Can you work these out from the drawing? Everything is in mm from the part's minimum corner. A direction names the side the tool comes from. Round coordinates to 2 decimals unless told otherwise and drop trailing zeros. Write each loop counter-clockwise with the first axis right and the second up, starting at its lowest first coordinate (ties: lowest second). Pieces come first, ordered by that corner, then holes. Notation, with made-up numbers: (51.5, -25.75) -> (75.5, -25.75) arc R9 ccw to (75.5, -9.75) -> close; hole circle Ø11 at (5.25, -14). An arc over 180 degrees is marked (long way). Write item = value, one per line. Start each with the question number.
1) Imagine slicing it at B-B, the plane x = 75. Please give me the cut outline in (y, z) (1 decimal).
2) Imagine slicing it at C-C, the plane y = 5.5. Please give me the cut outline in (x, z), then the cut area to 3 significant figures.
3) For the marked faces 1 and 2, which set-ups out of +Z, -Z, +X, -X, +Y, -Y let a thin tool reach every point of the face, with its end or its side?
4) Imagine slicing it at A-A, the plane z = 8. Please give me the cut outline in (x, y) (1 decimal).
5) If I drill on line 1 (Y direction, x = 52, z = 19) (1 decimal); line 2 (Z direction, x = 88.5, y = 21.5) (1 decimal); line 3 (Z direction, x = 17, y = 22), over which ranges is the centre line in solid material (lowest first)?
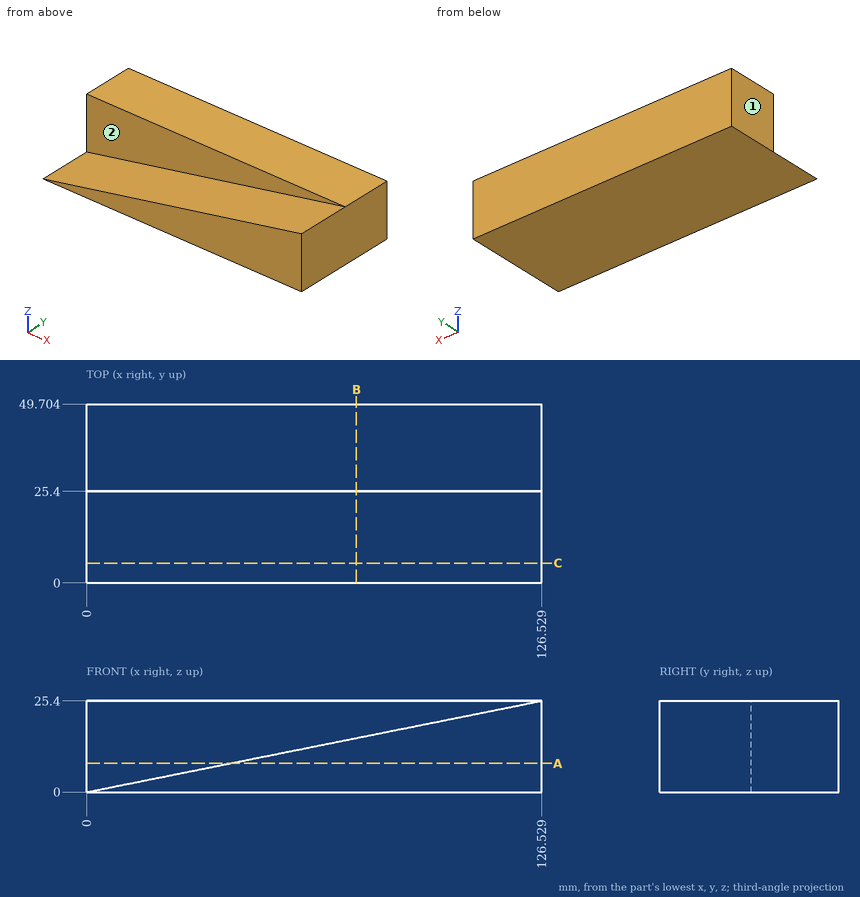
Reported:
q1.outline = (0, 0) -> (49.7, 0) -> (49.7, 25.4) -> (25.4, 25.4) -> (25.4, 15.1) -> (0, 15.1) -> close
q2.outline = (0, 0) -> (126.53, 0) -> (126.53, 25.4) -> close
q2.area = 1,610 mm²
q3.face_1 = +Z, -Z, -X, +Y, -Y
q3.face_2 = +Z, -X, -Y
q4.outline = (0, 25.4) -> (39.9, 25.4) -> (39.9, 0) -> (126.5, 0) -> (126.5, 49.7) -> (0, 49.7) -> close
q5.line_1 = 25.4 to 49.7
q5.line_2 = 0 to 17.8
q5.line_3 = 0 to 3.41
